```python
from build123d import *

# Parameters (mm, degrees)
F1_DEPTH  = 30
F2_W      = 10
F2_H      = 50
F3_DEPTH  = 7
F4_W      = 10
F4_H      = 8
F5_DEPTH  = 3.6
F8_DEPTH  = 26.5
F10_DEPTH = 8
F11_R     = 1.3
F12_DEPTH = 6
F13_R     = 1
F14_R     = 1.4
F16_DEPTH = 5
F15_R     = 1.4
F17_DEPTH = 5
F18_R     = 3
F19_R     = 4
F20_SIZE  = 1


with BuildPart() as f1:
    # F0 (on Front) → F1 (new body)
    with BuildSketch(Plane.XZ):
        Polygon((0, 32), (0, 0), (28, 0), (25.777778, 5), (20, 5), (8, 32), align=None)
    extrude(amount=F1_DEPTH)

    # F2 (on face) → F3 (join)
    with BuildSketch(Plane.XY.offset(32)):
        with Locations((5, -5)):
            Rectangle(F2_W, F2_H)
    extrude(amount=-F3_DEPTH)

    # F4 (on face) → F5 (cut)
    with BuildSketch(Plane.XY.offset(32)):
        with Locations((5, 14)):
            Rectangle(F4_W, F4_H)
        with Locations((5, -23.6)):
            Rectangle(F4_W, F4_H)
    extrude(amount=-F5_DEPTH, mode=Mode.SUBTRACT)

    # F7 (on offset) → F8 (cut)
    with BuildSketch(Plane.XZ.offset(28.25)):
        Polygon((18.891857, 3.8), (8.580746, 27), (7.580746, 27), (7.580746, 1.5), (22.944444, 1.5), (24.5, -2), (27.5, -2), (24.922222, 3.8), align=None)
    extrude(amount=-F8_DEPTH, mode=Mode.SUBTRACT)

    # F9 (on face) → F10 (cut)
    with BuildSketch(Plane(origin=(0, 0, 0), x_dir=(0, -1, 0), z_dir=(-1, 0, 0))):
        with BuildLine():
            Line((22.826238, 26), (7.173762, 26))
            ThreePointArc((7.173762, 26), (15, 1.5), (22.826238, 26))
        make_face()
    extrude(amount=-F10_DEPTH, mode=Mode.SUBTRACT)

    # F11 (on face) → F12 (cut)
    with BuildSketch(Plane(origin=(0, 0, 0), x_dir=(0, -1, 0), z_dir=(-1, 0, 0))):
        with Locations((3, 27)):
            Circle(F11_R)
        with Locations((3, 3)):
            Circle(F11_R)
        with Locations((27, 3)):
            Circle(F11_R)
    extrude(amount=-F12_DEPTH, mode=Mode.SUBTRACT)

    # F13
    f13_edges = [f1.edges().sort_by_distance(p)[0] for p in [
        (15, -30, 16.25),
        (15, 0, 16.25),
        (26.888889, -30, 2.5),
        (22.888889, -30, 5),
        (26.888889, 0, 2.5),
        (22.888889, 0, 5),
        (25.777778, -15, 5),
        (20, -15, 5),
        (14, -30, 0),
        (14, 0, 0),
    ]]
    fillet(f13_edges, radius=F13_R)

    # F14 (on face) → F16 (cut)
    with BuildSketch(Plane.XY.offset(28.4)):
        with Locations((3, 14.5)):
            Circle(F14_R)
    extrude(amount=-F16_DEPTH, mode=Mode.SUBTRACT)

    # F15 (on face) → F17 (cut)
    with BuildSketch(Plane.XY.offset(28.4)):
        with Locations((3, -24)):
            Circle(F15_R)
    extrude(amount=-F17_DEPTH, mode=Mode.SUBTRACT)

    # F18
    f18_edges = [f1.edges().sort_by_distance(p)[0] for p in [
        (18.891857, -15, 3.8),
    ]]
    fillet(f18_edges, radius=F18_R)

    # F19
    f19_edges = [f1.edges().sort_by_distance(p)[0] for p in [
        (24.922222, -15, 3.8),
    ]]
    fillet(f19_edges, radius=F19_R)

    # F20
    f20_edges = [f1.edges().sort_by_distance(p)[0] for p in [
        (22.944444, -15, 1.5),
    ]]
    chamfer(f20_edges, length=F20_SIZE)


solid = f1.part
```
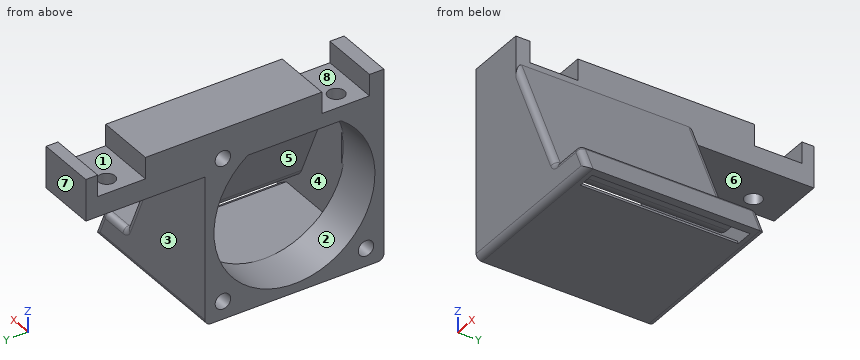
Design review of the part built by this model. Coordinates are the model's own, in mm. Face numbers are marked on the shaded views. A direction names the side the tool comes from. Give positions to 0.01 mm unless a question says otherwise; leave off trailing zeros. Write each loop counter-clockwise with the first axis right and the second up, starting at its lowest first coordinate (ties: lowest second). Pieces come first, ordered by that corner, then holes. Notation, with made-up numbers: (85, 29.25) - (129, 29.25) arc R27 cw to (129, 56.25) - close; hole circle Ø1 at (-39.75, 22.5). An arc over 180 degrees is marked (long way). Return JSON: item names as keys, results as strings. Group by question number.
(1) Machinability: for the marked faces 1, 2, 3 and 4, which of the approach directions +Z, -Z, +X, -X, +Y, -Y give a long, thin tool a straight path to every point of the face, cutting with its end or side? Answer none if there is none.
(2) We need section C-C, the plane y = -27. Give the boundary of the cut face in (x, z), then the cut area to 3 significant figures.
(3) We need section B-B, the plane y = 14.5. Give the boundary of the cut face in (x, z), then the cut area to 3 significant figures.
(4) Mouldability with a two-part tool opening along Y and no side actions: class the marked faces 5, 6, 7 and 8 as +Y half, -Y half, draft (parallel to the pull), parting line (faces both ways), or undercut.
(5) We need section A-A, the plane x = 3. Give the boundary of the cut face in (y, z), then the cut area to 3 significant figures.
(6) To check wall thickness, follow probe 1 along Y at (x, z) = (10.5, 22); probe 2 along Z at (x, y) = (5.75, -15); probe 3 along Z at (x, y) = (4.7, -3). State the ranges of each line that lie inside material, in increasing order.
(7) Insertion check: pin 1 (6 mm diameter, centred on y = -0.5, z = 25, fed in from +X); pin 2 (9.5 mm diameter, centred on x = 13.5, z = 7, fed in from +Y); pin 3 (5 mm diameter, centred on x = 6, y = 13, fed in from -Z). Each pin has a flat end and moves straight along its axis. Give the tip position at first contact, or say it passes through.
Reported:
{
 "1": {"face 1": "+Z, +X, -X", "face 2": "-X", "face 3": "-Z, +X, -X, +Y", "face 4": "none"},
 "2": {"outline": "(0, 0) - (23.61, 0) - (23.35, 0.59) - (21.94, 1.5) - (7.58, 1.5) - (7.58, 8.82) - (0, 8.82) - (0, 4.3) - (6, 4.3) - (6, 1.7) - (0, 1.7) - close; (0, 21.18) - (7.58, 21.18) - (7.58, 27) - (8.58, 27) - (18.1, 5.58) arc R3 ccw to (20.84, 3.8) - (22.32, 3.8) arc R4 cw to (25.98, 1.42) - (26.61, 0) - (28, 0) - (26.04, 4.41) arc R1 ccw to (25.13, 5) - (20.65, 5) arc R1 cw to (19.74, 5.59) - (10, 27.5) - (10, 28.4) - (0, 28.4) - close", "area": "183 mm2"},
 "3": {"outline": "(0, 25) - (1.6, 25) - (1.6, 28.4) - (0, 28.4) - close; (4.4, 25) - (10, 25) - (10, 28.4) - (4.4, 28.4) - close", "area": "24.5 mm2"},
 "4": {"face 5": "undercut", "face 6": "draft", "face 7": "+Y half", "face 8": "undercut"},
 "5": {"outline": "(-30, 1) arc R1 ccw to (-29, 0) - (-1, 0) arc R1 ccw to (0, 1) - (0, 25) - (13.1, 25) - (13.1, 28.4) - (10, 28.4) - (10, 32) - (-19.6, 32) - (-19.6, 28.4) - (-22.6, 28.4) - (-22.6, 26) - (-7.17, 26) arc R13.5 cw (long way) to (-25.4, 23.61) - (-25.4, 28.4) - (-27.6, 28.4) - (-27.6, 32) - (-30, 32) - close; (15.9, 25) - (20, 25) - (20, 32) - (18, 32) - (18, 28.4) - (15.9, 28.4) - close; hole circle Ø2.6 at (-27, 3); hole circle Ø2.6 at (-3, 3); hole circle Ø2.6 at (-3, 27)", "area": "461 mm2"},
 "6": {"probe 1": "y = -30 to -28.25, -1.75 to 0", "probe 2": "z = 0 to 1.5, 26 to 32", "probe 3": "z = 0 to 1.7, 4.3 to 8.82, 21.18 to 25.7, 28.3 to 32"},
 "7": {"pin 1": "stops at x = 12.43", "pin 2": "stops at y = 0", "pin 3": "stops at z = 25"}
}
